```python
from build123d import *

# Parameters (mm, degrees)
SKETCH_W      = 20
SKETCH_H      = 22
PAD_DEPTH     = 1
PAD001_DEPTH  = 3
SKETCH002_R   = 2.75
SKETCH002_W   = 18
SKETCH002_H   = 15
SKETCH002_W_2 = 7
SKETCH002_H_2 = 8
PAD002_DEPTH  = 3


with BuildPart() as part:
    # Sketch → Pad (new body)
    with BuildSketch(Plane.XY):
        with Locations((0, 11)):
            Rectangle(SKETCH_W, SKETCH_H)
    extrude(amount=PAD_DEPTH)

    # Sketch001 (on Face6 of Pad) → Pad001 (join)
    with BuildSketch(Plane.XY.offset(1)):
        with BuildLine():
            Line((-7, 20), (7, 20))
            ThreePointArc((9, 18), (8.414214, 19.414214), (7, 20))
            Line((9, 18), (9, 4))
            ThreePointArc((7, 2), (8.414214, 2.585786), (9, 4))
            Line((-7, 2), (7, 2))
            ThreePointArc((-9, 4), (-8.414214, 2.585786), (-7, 2))
            Line((-9, 18), (-9, 4))
            Line((-9, 18), (-7, 20))
        make_face()
    extrude(amount=PAD001_DEPTH)

    # Sketch002 (on Face4 of Pad001) → Pad002 (join)
    with BuildSketch(Plane(origin=(0, 0, 0), x_dir=(1, 0, 0), z_dir=(0, 0, -1))):
        with Locations((-6.7, -3.1)):
            Circle(SKETCH002_R)
        with Locations((0, -13.7)):
            Rectangle(SKETCH002_W, SKETCH002_H)
        Rectangle(SKETCH002_W_2, SKETCH002_H_2)
    extrude(amount=PAD002_DEPTH)


solid = part.part
```
The listing builds one solid part. Answer for the finished solid, in the listing's coordinates (mm). A direction names the side the tool comes from. Coordinates: 2 decimals unless noted, no trailing zeros. Write each loop counter-clockwise with the first axis right and the second up, starting at its lowest first coordinate (ties: lowest second). Pieces come first, ordered by that corner, then holes. Notation, with made-up numbers: (-16, -30) - (36, -30) arc R31 cw to (36, -4) - close; hole circle Ø10 at (7.25, -0.5). An arc over 180 degrees is marked (long way). Return JSON: item names as keys, results as strings. Group by question number.
Q1. The part is cut by section B-B on y = 9. Write down the section's boundary in (x, z).
Q2. Flat-ended cylindrical pins translate along their axes: pin 1 Ø0.9 at (y, z) = (12.5, 2.5) entering from +X; pin 2 Ø1.5 at (x, z) = (4.5, -2) entering from +Y; pin 3 Ø1.5 at (y, z) = (3.5, -2) entering from +X; pin 4 Ø4 at (y, z) = (-0.5, 3) entering from +X. Find the tip coordinate at first contact, or state that the pin passes through.
Q3. The part is cut by section D-D on x = 2.25. Write down the section's boundary in (y, z), and give its area (3 significant figures).
Q4. The part is cut by section A-A on z = -1. Write down the section's boundary in (x, y), and give its area (3 significant figures).
Q5. For a pull along X with two mould halves and no side action, classify faces 1 (the flat face through (0, 2, 2)), 2 (the flat face through (9, 14, -1)), 3 (the cylindrical face through (-8.882, 4.773, -1.479)), 4 (the flat face through (-10, 10.8, 0.5)) as +X half, -X half, draft (parallel to the pull), parting line (faces both ways), or undercut.
Q6. Which of the six approach directions +Z, -Z, +X, -X, +Y, -Y give full straight-line access (tool end or side, diameter ignored) to faces 5 (the cylindrical face through (8.4, 2.57, 2.48)), 6 (the flat face through (-9, 14, -1)), 7 (the flat face through (0, 21.2, -1)), 8 (the flat face through (-0.1, 0, 0.5))?
Q7. The part is cut by section C-C on x = -6.7. Write down the section's boundary in (y, z).
Q8. Find the intervals of material crossed by line 1 along Y through (x, z) = (2.25, -0.75); line 2 along X through (y, z) = (11, -1.25); line 3 along Z through (x, y) = (8.5, 5.5), in increasing order. Write a range as [from, to].
Evaluation:
{
 "1": {"outline": "(-10, 0) - (-9, 0) - (-9, -3) - (9, -3) - (9, 0) - (10, 0) - (10, 1) - (9, 1) - (9, 4) - (-9, 4) - (-9, 1) - (-10, 1) - close"},
 "2": {"pin 1": "stops at x = 9", "pin 2": "stops at y = 21.2", "pin 3": "stops at x = 3.5", "pin 4": "passes through"},
 "3": {"outline": "(-4, -3) - (4, -3) - (4, 0) - (6.2, 0) - (6.2, -3) - (21.2, -3) - (21.2, 0) - (22, 0) - (22, 1) - (20, 1) - (20, 4) - (2, 4) - (2, 1) - (0, 1) - (0, 0) - (-4, 0) - close", "area": "145 mm2"},
 "4": {"outline": "circle Ø5.5 at (-6.7, 3.1); (-9, 6.2) - (9, 6.2) - (9, 21.2) - (-9, 21.2) - close; (-3.5, -4) - (3.5, -4) - (3.5, 4) - (-3.5, 4) - close", "area": "350 mm2"},
 "5": {"face 1": "draft", "face 2": "+X half", "face 3": "undercut", "face 4": "-X half"},
 "6": {"face 5": "+Z, +X, -Y", "face 6": "-Z, -X, +Y", "face 7": "-Z, +X, -X, +Y", "face 8": "+Z, +X, -X, -Y"},
 "7": {"outline": "(0, 0) - (0.35, 0) - (0.35, -3) - (5.85, -3) - (5.85, 0) - (6.2, 0) - (6.2, -3) - (21.2, -3) - (21.2, 0) - (22, 0) - (22, 1) - (20, 1) - (20, 4) - (2, 4) - (2, 1) - (0, 1) - close"},
 "8": {"line 1": "y = [-4, 4], [6.2, 21.2]", "line 2": "x = [-9, 9]", "line 3": "z = [0, 4]"}
}
